Print and shaded views of the part. All mm, measured from the part's lowest x, y and z. Round coordinates to 2 decimals unless told otherwise and drop trailing zeros. Order: outer loops, then holes, each group sorted by start corner. A loop starts at its lowest first (then second) coordinate and runs counter-clockwise, first axis right, second up. Notation, with made-up numbers: (73.5, 6) - (95.5, 6) arc R20 ccw to (95.5, 28) - close; hole circle Ø2 at (24.25, 51). An arc over 180 degrees is marked (long way). Return JSON: item names as keys, results as strings. Group by question number.
Item 1: Saw through at A-A on y = 3.35. List the corners of the cut face in (x, z).
Item 2: Saw through at B-B on x = 2. List the corners of the cut face in (y, z).
Item 3: Probe probe 1 along X at (y, z) = (3.6, 16.75); probe 2 along X at (y, z) = (1.45, 1.75); probe 3 along Z at (x, y) = (2, 2.9). List the from-to ranges inside material, lowest first.
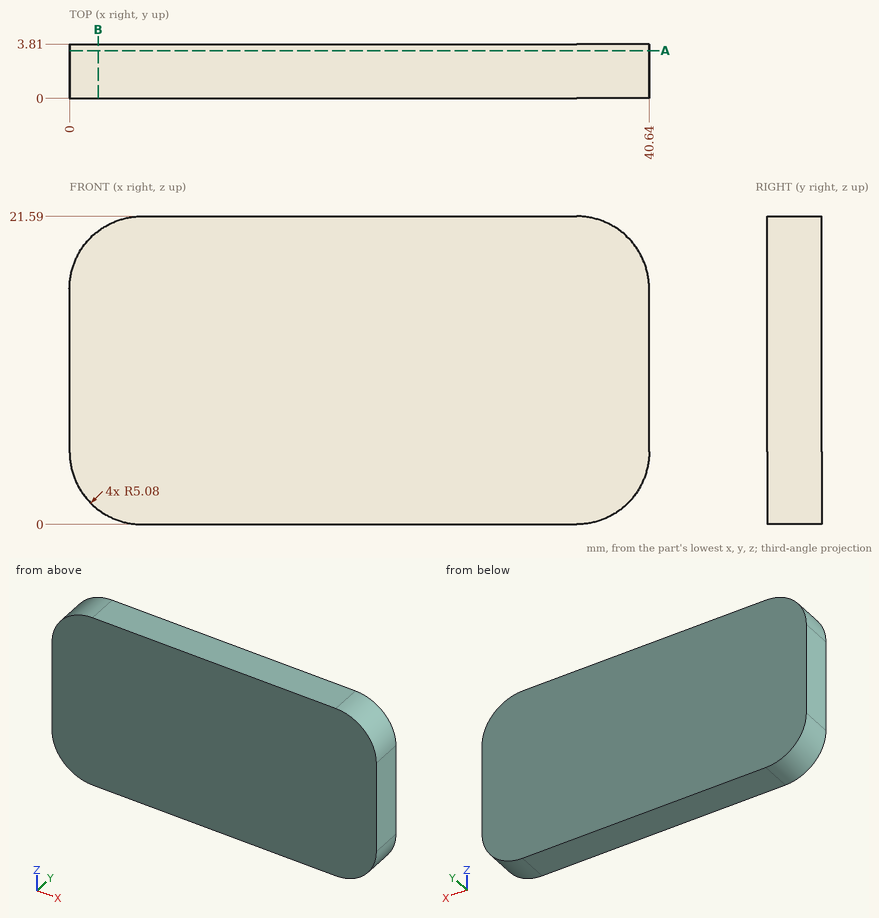
Filled in:
{
 "1": {"outline": "(0, 5.08) arc R5.08 ccw to (5.08, 0) - (35.56, 0) arc R5.08 ccw to (40.64, 5.08) - (40.64, 16.51) arc R5.08 ccw to (35.56, 21.59) - (5.08, 21.59) arc R5.08 ccw to (0, 16.51) - close"},
 "2": {"outline": "(0, 1.04) - (3.81, 1.04) - (3.81, 20.55) - (0, 20.55) - close"},
 "3": {"probe 1": "x = 0.01 to 40.63", "probe 2": "x = 1.24 to 39.4", "probe 3": "z = 1.04 to 20.55"}
}
